Check sheet for the modelled part. Datum: model origin and axes. Units: mm. Coordinates: 2 decimals unless noted, no trailing zeros. Loops run counter-clockwise (first coordinate to the right, second up) from the corner with the lowest first, then second, coordinate; pieces in that order, holes last. Notation, with made-up numbers: (-1.5, 63) -> (4.5, 63) arc R21 cw to (4.5, 92) -> close; hole circle Ø11 at (-9, 89). An arc over 180 degrees is marked (long way). Use CSV: the item, a comma, the result in double quotes. Start each with the question number.
1. Sectioned sample at D-D, the plane x = -48.5. Record the cut outline in (y, z), and give its area (3 significant figures).
2. Sectioned sample at A-A, the plane y = 0. Record the cut outline in (x, z).
3. Sectioned sample at B-B, the plane x = -15. Record the cut outline in (y, z), and give its area (3 significant figures).
4. Sectioned sample at C-C, the plane z = 29. Record the cut outline in (x, y), and give its area (3 significant figures).
5. Gauge pin test, flat ends, axial feed: pin 1 (24.5 mm diameter, centred on x = -9.144, y = 0, fed in from +Z); pin 2 (4 mm diameter, centred on x = -25, z = 31.5, fed in from -Y). Record the tip position at first contact, or that the pin passes through.
6. Thickness scan on L1, parallel to X at y = -3, z = 5; L2, parallel to Y at x = -21.5, z = 46.5; L3, parallel to Y at x = -2.5, z = 32. Record the ranges inside material, lowest first.
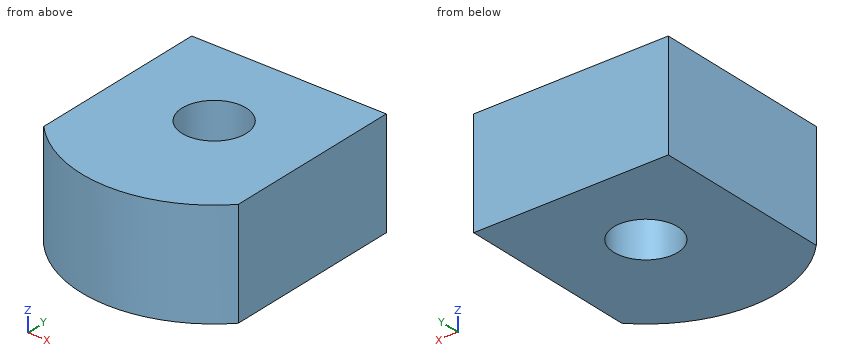
```python
from build123d import *

# Parameters (mm, degrees)
F0_W     = 92.964003
F0_H     = 87.376002
F0_R     = 15.291068
F1_DEPTH = 50.8


with BuildPart() as f1:
    # F0 (on Top) → F1 (new body)
    with BuildSketch(Plane.XY):
        with Locations((-9.143999, 0.505356)):
            Rectangle(F0_W, F0_H)
        with Locations((-9.144, 0)):
            Circle(F0_R, mode=Mode.SUBTRACT)
        with BuildLine():
            Line((37.338002, -43.182645), (-55.626001, -43.182645))
            ThreePointArc((-55.626001, -43.182645), (-9.144, -63.445388), (37.338002, -43.182645))
        make_face()
    extrude(amount=F1_DEPTH)


solid = f1.part
```
Completed:
1,outline,"(-49.76, 0) -> (44.19, 0) -> (44.19, 50.8) -> (-49.76, 50.8) -> close"
1,area,"4,770 mm²"
2,outline,"(-55.63, 0) -> (-24.44, 0) -> (-24.44, 50.8) -> (-55.63, 50.8) -> close; (6.15, 0) -> (37.34, 0) -> (37.34, 50.8) -> (6.15, 50.8) -> close"
3,outline,"(-63.17, 0) -> (-14.13, 0) -> (-14.13, 50.8) -> (-63.17, 50.8) -> close; (14.13, 0) -> (44.19, 0) -> (44.19, 50.8) -> (14.13, 50.8) -> close"
3,area,"4,020 mm²"
4,outline,"(-55.63, -43.18) arc R63.45 ccw to (37.34, -43.18) -> (37.34, 44.19) -> (-55.63, 44.19) -> close; hole circle Ø30.58 at (-9.14, 0)"
4,area,"8,690 mm²"
5,pin 1,"through"
5,pin 2,"y = -61.91"
6,L1,"-55.63 to -24.14, 5.85 to 37.34"
6,L2,"-62.23 to -9.01, 9.01 to 44.19"
6,L3,"-63.1 to -13.77, 13.77 to 44.19"
